Read the model definition and answer for the solid it produces. Units are mm, in the model's axes. Face numbers are marked on the shaded views. A direction names the side the tool comes from. Coordinates: 2 decimals unless noted, no trailing zeros. Write each loop counter-clockwise with the first axis right and the second up, starting at its lowest first coordinate (ties: lowest second). Pieces come first, ordered by that corner, then holes. Notation, with made-up numbers: (64.5, -8) -> (108.5, -8) arc R16 cw to (108.5, 5) -> close; hole circle Ø11 at (-28.75, 51.25). An arc over 180 degrees is marked (long way). Answer as a JSON object with one key per item and string values. Group by question number.
(1) For a pull along X with two mould halves and no side action, classify the marked faces 6, 7, 8 and 9 as +X half, -X half, draft (parallel to the pull), parting line (faces both ways), or undercut.
(2) Which of the six approach directions +Z, -Z, +X, -X, +Y, -Y give full straight-line access (tool end or side, diameter ignored) to the marked faces 1, 2, 3, 4 and 5?
(3) Straight lines are drawn through the part: L1, parallel to Y at x = 0, z = -3.4; L2, parallel to X at y = -9.75, z = 0.25; L3, parallel to X at y = -7.5, z = -3.05. For each, find the intervals that lie inside material, in ascending order.
(4) Find section C-C (y = -7.5). Give the vertices of the cut face in (x, z).
(5) Find section A-A (y = -15.5). Give the vertices of the cut face in (x, z), then the cut area to 3 significant figures.
(6) Find section B-B (z = -2.75). Give the vertices of the cut face in (x, y), then the cut area to 3 significant figures.
(7) Flat-ended cylindrical pins translate along their axes: P1, Ø1.5, axis at x = -2.5, z = 1.5, coming from the -Y side; P2, Ø1.5, axis at x = 0, y = -7.5, coming from the -Z side; P3, Ø0.6, axis at x = 0, y = -28, coming from the +Z side. Find the tip coordinate at first contact, or state that the pin passes through.
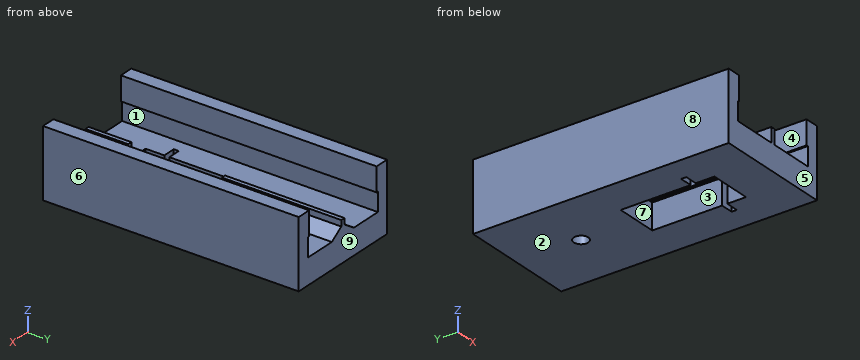
from build123d import *

# Parameters (mm, degrees)
F0_W     = 14
F0_H     = 8
F1_DEPTH = 30
F3_W     = 1.5
F3_H     = 0.6
F4_DEPTH = 8
F5_DEPTH = 30.001
F7_DEPTH = 5
F8_R     = 0.85
F9_DEPTH = 3


# Not quite as in the source:
# - a feature names something its author has since deleted; it is built from what else it names


with BuildPart() as f1:
    # F0 (on Front) → F1 (new body)
    with BuildSketch(Plane.XZ):
        Rectangle(F0_W, F0_H)
    extrude(amount=F1_DEPTH)

    # F3 (on face) → F4 (cut, through all)
    with BuildSketch(Plane(origin=(0, 0, -4), x_dir=(1, 0, 0), z_dir=(0, 0, -1))):
        with Locations((3.25, 22.5)):
            Rectangle(F3_W, F3_H)
        Polygon((-2.5, 14), (2.5, 14), (2.5, 22.2), (2.5, 22.8), (2.5, 25), (-2.5, 25), (-2.5, 22.8), (-2.5, 22.2), align=None)
        with Locations((-3.25, 22.5)):
            Rectangle(F3_W, F3_H)
    extrude(amount=-F4_DEPTH, mode=Mode.SUBTRACT)

    # F2 (on face) → F5 (cut, through all)
    with BuildSketch(Plane.XZ.offset(30)):
        Polygon((-0.25, 0), (-0.25, 0.7), (0.25, 0.7), (0.25, 0), (1.75, -1), (5.55, -1), (5.55, 1.2), (5.35, 1.2), (5.35, 4), (-5.35, 4), (-5.35, 1.2), (-5.55, 1.2), (-5.55, -1), (-1.75, -1), align=None)
    extrude(amount=-F5_DEPTH, mode=Mode.SUBTRACT)

    # F6 (on face) → F7 (cut, through all)
    with BuildSketch(Plane.XZ.offset(30)):
        Polygon((-0.25, -1), (-0.25, 0), (-1.75, -1), align=None)
        Polygon((1.75, -1), (0.25, 0), (0.25, -1), align=None)
    extrude(amount=-F7_DEPTH, mode=Mode.SUBTRACT)

    # F8 (on face) → F9 (cut)
    with BuildSketch(Plane(origin=(0, 0, -4), x_dir=(1, 0, 0), z_dir=(0, 0, -1))):
        with Locations((0, 7.5)):
            Circle(F8_R)
    extrude(amount=-F9_DEPTH, mode=Mode.SUBTRACT)


solid = f1.part
Results below:
{
 "1": {"face 6": "+X half", "face 7": "undercut", "face 8": "-X half", "face 9": "draft"},
 "2": {"face 1": "+Y, -Y", "face 2": "-Z, +X, -X, +Y, -Y", "face 3": "+Z, -Z", "face 4": "+Z, +Y, -Y", "face 5": "+Z, -Z, +X, -X, -Y"},
 "3": {"L1": "y = -30 to -25, -14 to -8.35, -6.65 to 0", "L2": "x = -7 to -5.55, -0.25 to 0.25, 5.55 to 7", "L3": "x = -7 to -0.85, 0.85 to 7"},
 "4": {"outline": "(-7, -4) -> (-0.85, -4) -> (-0.85, -1) -> (0.85, -1) -> (0.85, -4) -> (7, -4) -> (7, 4) -> (5.35, 4) -> (5.35, 1.2) -> (5.55, 1.2) -> (5.55, -1) -> (1.75, -1) -> (0.25, 0) -> (0.25, 0.7) -> (-0.25, 0.7) -> (-0.25, 0) -> (-1.75, -1) -> (-5.55, -1) -> (-5.55, 1.2) -> (-5.35, 1.2) -> (-5.35, 4) -> (-7, 4) -> close"},
 "5": {"outline": "(-7, -4) -> (-2.5, -4) -> (-2.5, -1) -> (-5.55, -1) -> (-5.55, 1.2) -> (-5.35, 1.2) -> (-5.35, 4) -> (-7, 4) -> close; (2.5, -4) -> (7, -4) -> (7, 4) -> (5.35, 4) -> (5.35, 1.2) -> (5.55, 1.2) -> (5.55, -1) -> (2.5, -1) -> close", "area": "42.6 mm2"},
 "6": {"outline": "(-7, -30) -> (7, -30) -> (7, 0) -> (-7, 0) -> close; hole (-4, -22.8) -> (-2.5, -22.8) -> (-2.5, -25) -> (2.5, -25) -> (2.5, -22.8) -> (4, -22.8) -> (4, -22.2) -> (2.5, -22.2) -> (2.5, -14) -> (-2.5, -14) -> (-2.5, -22.2) -> (-4, -22.2) -> close; hole circle Ø1.7 at (0, -7.5)", "area": "361 mm2"},
 "7": {"P1": "passes through", "P2": "stops at z = -1", "P3": "stops at z = 0.7"}
}
